from build123d import *

# Parameters (mm, degrees)
SKETCH1_W           = 285
SKETCH1_H           = 170
BOSS_EXTRUDE1_DEPTH = 12
SKETCH2_R           = 2.5
SKETCH4_W           = 60
SKETCH4_H           = 30
BOSS_EXTRUDE2_DEPTH = 3
CUT_EXTRUDE1_DEPTH  = 195.554619595


with BuildPart() as part:
    # Sketch1 → Boss-Extrude1 (new body)
    with BuildSketch(Plane(origin=(0, 0, 0), x_dir=(1, 0, 0), z_dir=(0, 1, 0))):
        Rectangle(SKETCH1_W, SKETCH1_H)
    extrude(amount=BOSS_EXTRUDE1_DEPTH)

    # Sweep1: sweep along a path in Sketch3
    with BuildLine(Plane.XY) as sweep1_path:
        Line((-50, 12), (-50, 32))
        ThreePointArc((-50, 32), (-47.071067812, 39.071067812), (-40, 42))
        Line((-40, 42), (40, 42))
        ThreePointArc((40, 42), (47.071067812, 39.071067812), (50, 32))
        Line((50, 32), (50, 12))
    # Sketch2 → Sweep1 (sweep)
    with BuildSketch(Plane(origin=(0, 12, 0), x_dir=(1, 0, 0), z_dir=(0, 1, 0))):
        with Locations((-50, 0)):
            Circle(SKETCH2_R)
    sweep(path=sweep1_path.line)

    # Sketch4 → Boss-Extrude2 (add)
    with BuildSketch(Plane(origin=(0, 12, 0), x_dir=(1, 0, 0), z_dir=(0, 1, 0))):
        with Locations((142.5, -58)):
            Rectangle(SKETCH4_W, SKETCH4_H)
        with Locations((-142.5, -58)):
            Rectangle(SKETCH4_W, SKETCH4_H)
    extrude(amount=BOSS_EXTRUDE2_DEPTH)

    # Sketch5 → Cut-Extrude1 (cut, symmetric)
    with BuildSketch(Plane(origin=(0, 15, 0), x_dir=(1, 0, 0), z_dir=(0, 1, 0))):
        with BuildLine():
            Line((157.5, -64.5), (172.5, -64.5))
            Line((172.5, -64.5), (172.5, -51.5))
            Line((172.5, -51.5), (157.5, -51.5))
            ThreePointArc((157.5, -51.5), (151, -58), (157.5, -64.5))
        make_face()
    cut_extrude1 = extrude(amount=CUT_EXTRUDE1_DEPTH, both=True, mode=Mode.SUBTRACT)

    # Mirror1: Cut-Extrude1 across plane
    add(cut_extrude1.mirror(Plane(origin=(0, 0, 0), x_dir=(0, 0, 1), z_dir=(1, 0, 0))), mode=Mode.SUBTRACT)


solid = part.part
Work out the finished part from the listing and answer in its coordinate system (mm). A direction names the side the tool comes from. Round coordinates to 2 decimals unless told otherwise and drop trailing zeros. Write each loop counter-clockwise with the first axis right and the second up, starting at its lowest first coordinate (ties: lowest second). Pieces come first, ordered by that corner, then holes.
1) A cutting plane is placed at D-D (x = 125.5). Give the vertices of the cut face in (y, z), plus the area to 3 significant figures.
2) A cutting plane is placed at C-C (y = 7). Give the vertices of the cut face in (x, z).
3) Straight lines are drawn through the part: line 1 (X direction, y = 8.5, z = -21); line 2 (Y direction, x = 12, z = -7); line 3 (Y direction, x = -150, z = 62.5). For each, find the intervals that lie inside material, in ascending order.
4) A cutting plane is placed at A-A (x = 27). Give the vertices of the cut face in (y, z), plus the area to 3 significant figures.
5) The mould has two halves that part along Z. Classify faces 1 (the cylindrical face through (151, 14, 58)), 2 (the flat face through (-2, 6, -85)), 3 (the flat face through (-143, 15, 58)): pulls with the +Z half, pulls with the -Z half, needs draft (parallel to the pull), parting line crosses it, or undercut.
6) Given pin 1 Ø2.5 at (x, y) = (168.5, 13.5) entering from +Z; pin 2 Ø10 at (x, z) = (100, 59) entering from +Y; pin 3 Ø8 at (y, z) = (14.5, 59.5) entering from -X, each flat-ended and moving along its own axis, determine where each tip first touches the part or whether it passes through.
7) A tool of negligible diameter and unlimited length cuts with its end or side. For faces 4 (the flat face through (150.6, 12, 57.8)), 5 (the flat face through (-2, 6, 85)), 6 (the flat face through (-151, 12, 54)), from which of +Z, -Z, +X, -X, +Y, -Y can it reach the whole face along a straight path? Write none if from no direction.
8) A cutting plane is placed at B-B (z = 58). Give the vertices of the cut face in (x, y), plus the area to 3 significant figures.
Completed:
1. outline: (0, -85) - (12, -85) - (12, 43) - (15, 43) - (15, 73) - (12, 73) - (12, 85) - (0, 85) - close
1. area: 2,130 mm2
2. outline: (-142.5, -85) - (142.5, -85) - (142.5, 85) - (-142.5, 85) - close
3. line 1: x = -142.5 to 142.5
3. line 2: y = 0 to 12
3. line 3: y = 12 to 15
4. outline: (0, -85) - (12, -85) - (12, 85) - (0, 85) - close; circle Ø5 at (42, 0)
4. area: 2,060 mm2
5. face 1: undercut
5. face 2: pulls with the -Z half
5. face 3: needs draft
6. pin 1: stops at z = 73
6. pin 2: stops at y = 12
6. pin 3: stops at x = -154.04
7. face 4: +Z, -Z, +X, -Y
7. face 5: +Z, +X, -X, +Y, -Y
7. face 6: +Z, -Z, -X, -Y
8. outline: (-151, 12) - (-142.5, 12) - (-142.5, 0) - (142.5, 0) - (142.5, 12) - (151, 12) - (151, 15) - (112.5, 15) - (112.5, 12) - (-112.5, 12) - (-112.5, 15) - (-151, 15) - close
8. area: 3,650 mm2
